```python
from build123d import *

# Parameters (mm, degrees)
F1_DEPTH = 2.5
F0_W     = 13
F0_H     = 38.5
F2_DEPTH = 1
F4_DEPTH = 1


with BuildPart() as f1:
    # F0 (on Front) → F1 (new body)
    with BuildSketch(Plane.XZ):
        Polygon((-11.071428, 40), (-11.071428, 0), (-9.571428, 0), (-9.571428, 38.5), (3.428572, 38.5), (3.428572, 0), (4.928572, 0), (4.928572, 40), align=None)
    extrude(amount=F1_DEPTH)

    # F0 (on Front) → F2 (join)
    with BuildSketch(Plane.XZ):
        with Locations((-3.071428, 19.25)):
            Rectangle(F0_W, F0_H)
    extrude(amount=F2_DEPTH)

    # F3 (on face) → F4 (join)
    with BuildSketch(Plane.XZ.offset(1)):
        with BuildLine():
            Line((1.137349, 19), (-1.132357, 19))
            ThreePointArc((-1.132357, 19), (-1.632357, 18.5), (-1.132357, 18))
            Line((-1.132357, 18), (1.137349, 18))
            ThreePointArc((1.137349, 18), (1.637349, 18.5), (1.137349, 19))
        make_face()
    extrude(amount=F4_DEPTH)


solid = f1.part
```
Design review of the part built by this model. Coordinates are the model's own, in mm. A direction names the side the tool comes from. Round coordinates to 2 decimals unless told otherwise and drop trailing zeros. Write each loop counter-clockwise with the first axis right and the second up, starting at its lowest first coordinate (ties: lowest second). Pieces come first, ordered by that corner, then holes. Notation, with made-up numbers: (2.5, -39) -> (36.5, -39) arc R23 ccw to (36.5, -11) -> close; hole circle Ø6 at (-26, 50). An arc over 180 degrees is marked (long way). Write item = value, one per line. Start each with the question number.
1) Tool access review of faces 1 (the face through (-3, -2, 38.5)), 2 (the face through (-3, 0, 20)), 3 (the face through (-9.571, -2, 19)): name each direction out of +Z, -Z, +X, -X, +Y, -Y from which nothing blocks a thin tool from reaching the whole face with its end or side.
2) Take a section at D-D, the plane z = 9.5. State the section outline as (x, y) points.
3) Take a section at B-B, the plane z = 18.5. State the section outline as (x, y) points.
4) Take a section at A-A, the plane y = -1.5. State the section outline as (x, z) points.
5) Take a section at C-C, the plane x = -8. State the section outline as (y, z) points.
6) Clearance check with flat-ended pins moving along their axes: pin 1 (0.5 mm diameter, centred on x = 0.5, y = -1.5, fed in from -Z); pin 2 (0.8 mm diameter, centred on x = -0.5, z = 18.5, fed in from -Y); pin 3 (4 mm diameter, centred on x = -3, z = 22, fed in from -Y). State where each tip first meets the part, or that it passes through.
7) Mouldability with a two-part tool opening along Z and no side actions: class faces 4 (the face through (-3, -1, 40)), 5 (the face through (0, -1.5, 19)), 6 (the face through (0, -2, 18.5)) as +Z half, -Z half, draft (parallel to the pull), parting line (faces both ways), or undercut.
8) Wall thickness on probe 1 along X at (y, z) = (-2.4, 32.5); probe 2 along Z at (x, y) = (2, -2.3); probe 3 along Y at (x, z) = (0.5, 2): over which ranges is each line inside the solid? List them lowest first. Write a range as from..to.
Results list:
q1.face_1 = -Y
q1.face_2 = +Z, -Z, +X, -X, +Y
q1.face_3 = -Z, -Y
q2.outline = (-11.07, -2.5) -> (-9.57, -2.5) -> (-9.57, -1) -> (3.43, -1) -> (3.43, -2.5) -> (4.93, -2.5) -> (4.93, 0) -> (-11.07, 0) -> close
q3.outline = (-11.07, -2.5) -> (-9.57, -2.5) -> (-9.57, -1) -> (-1.63, -1) -> (-1.63, -2) -> (1.64, -2) -> (1.64, -1) -> (3.43, -1) -> (3.43, -2.5) -> (4.93, -2.5) -> (4.93, 0) -> (-11.07, 0) -> close
q4.outline = (-11.07, 0) -> (-9.57, 0) -> (-9.57, 38.5) -> (3.43, 38.5) -> (3.43, 0) -> (4.93, 0) -> (4.93, 40) -> (-11.07, 40) -> close; (-1.13, 18) -> (1.14, 18) arc R0.5 ccw to (1.14, 19) -> (-1.13, 19) arc R0.5 ccw to start
q5.outline = (-2.5, 38.5) -> (-1, 38.5) -> (-1, 0) -> (0, 0) -> (0, 40) -> (-2.5, 40) -> close
q6.pin_1 = 18
q6.pin_2 = -2
q6.pin_3 = -1
q7.face_4 = +Z half
q7.face_5 = undercut
q7.face_6 = draft
q8.probe_1 = -11.07..-9.57, 3.43..4.93
q8.probe_2 = 38.5..40
q8.probe_3 = -1..0
